from build123d import *

# Parameters (mm, degrees)
BOSS_EXTRU_1_DEPTH         = 3
CONG_1_R                   = 3
ESQUISSE2_R                = 3
PER_AGE_PROFIL_DEPTH       = 200.145675323
ESQUISSE3_R                = 1.65
PER_AGE_ENCODEUR_DEPTH     = 200.145675323
POCHE_ROUE_ENCODEUSE_DEPTH = 200.145675323
CONG_4_R                   = 1
CONG_2_R                   = 4.25
CONG_3_R                   = 4.25
ESQUISSE5_R                = 1.65
PER_AGE_BLOC_MOTEUR_DEPTH  = 200.145675323
ESQUISSE6_W                = 28
ESQUISSE6_H                = 68
POCHE_ROUE_MOTRICE_DEPTH   = 200.145675323
ESQUISSE7_R                = 3.5
PER_AGE_PATIN_DEPTH        = 200.145675323
ESQUISSE8_R                = 3
ENL_V_MAT_EXTRU_1_DEPTH    = 200.145675323
CONG_5_R                   = 6
ENL_V_MAT_EXTRU_2_REACH    = 201.146
ESQUISSE9_W                = 7.25
ESQUISSE9_H                = 65
CONG_6_R                   = 2
ESQUISSE10_R               = 1.75
ENL_V_MAT_EXTRU_3_DEPTH    = 200.145675323


with BuildPart() as part:
    # Esquisse1 → Boss.-Extru.1 (new body)
    with BuildSketch(Plane(origin=(0, 0, 0), x_dir=(1, 0, 0), z_dir=(0, 1, 0))):
        Polygon((-130, 125), (130, 125), (155, 100), (155, -100), (130, -125), (-130, -125), (-155, -100), (-155, 100), align=None)
    extrude(amount=BOSS_EXTRU_1_DEPTH)

    # Congé1
    cong_1_edges = [part.edges().sort_by_distance(p)[0] for p in [
        (155, 1.5, -100),
        (155, 1.5, 100),
        (130, 1.5, 125),
        (-130, 1.5, 125),
        (-155, 1.5, 100),
        (-155, 1.5, -100),
        (-130, 1.5, -125),
        (130, 1.5, -125),
    ]]
    fillet(cong_1_edges, radius=CONG_1_R)

    # Esquisse2 → Perçage Profilé (cut, through all)
    with BuildSketch(Plane(origin=(0, 3, 0), x_dir=(1, 0, 0), z_dir=(0, 1, 0))):
        with Locations(Location((-132, -65, 0), (0, 0, 270))):
            Circle(ESQUISSE2_R)
        with Locations(Location((-132, 65, 0), (0, 0, 90))):
            Circle(ESQUISSE2_R)
        with Locations(Location((132, -65, 0), (0, 0, 90))):
            Circle(ESQUISSE2_R)
        with Locations(Location((132, 65, 0), (0, 0, 270))):
            Circle(ESQUISSE2_R)
    extrude(amount=-PER_AGE_PROFIL_DEPTH, mode=Mode.SUBTRACT)

    # Esquisse3 → Perçage Encodeur (cut, through all)
    with BuildSketch(Plane(origin=(0, 3, 0), x_dir=(1, 0, 0), z_dir=(0, 1, 0))):
        with Locations(Location((-127, 19, 0), (0, 0, 270))):
            Circle(ESQUISSE3_R)
        with Locations(Location((-127, -19, 0), (0, 0, 270))):
            Circle(ESQUISSE3_R)
        with Locations(Location((127, -19, 0), (0, 0, 90))):
            Circle(ESQUISSE3_R)
        with Locations(Location((127, 19, 0), (0, 0, 90))):
            Circle(ESQUISSE3_R)
        with Locations(Location((-139.5, 31, 0), (0, 0, 270))):
            Circle(ESQUISSE3_R)
        with Locations(Location((-139.5, -31, 0), (0, 0, 270))):
            Circle(ESQUISSE3_R)
        with Locations(Location((139.5, -31, 0), (0, 0, 90))):
            Circle(ESQUISSE3_R)
        with Locations(Location((139.5, 31, 0), (0, 0, 90))):
            Circle(ESQUISSE3_R)
    extrude(amount=-PER_AGE_ENCODEUR_DEPTH, mode=Mode.SUBTRACT)

    # Esquisse4 → Poche Roue Encodeuse (cut, through all)
    with BuildSketch(Plane(origin=(0, 3, 0), x_dir=(1, 0, 0), z_dir=(0, 1, 0))):
        with BuildLine():
            Line((143.5, -15), (129.5, -15))
            ThreePointArc((129.5, -15), (128.792893219, -14.707106781), (128.5, -14))
            Line((128.5, -14), (128.5, 14))
            ThreePointArc((128.5, 14), (128.792893219, 14.707106781), (129.5, 15))
            Line((129.5, 15), (143.5, 15))
            Line((143.5, 15), (143.5, 32.5))
            Line((143.5, 32.5), (152, 32.5))
            Line((152, 32.5), (152, -32.5))
            Line((152, -32.5), (143.5, -32.5))
            Line((143.5, -32.5), (143.5, -15))
        make_face()
        with BuildLine():
            Line((-128.5, -14), (-128.5, 14))
            ThreePointArc((-128.5, 14), (-128.792893219, 14.707106781), (-129.5, 15))
            Line((-129.5, 15), (-143.5, 15))
            Line((-143.5, 15), (-143.5, 32.5))
            Line((-143.5, 32.5), (-152, 32.5))
            Line((-152, 32.5), (-152, -32.5))
            Line((-152, -32.5), (-143.5, -32.5))
            Line((-143.5, -32.5), (-143.5, -15))
            Line((-143.5, -15), (-129.5, -15))
            ThreePointArc((-129.5, -15), (-128.792893219, -14.707106781), (-128.5, -14))
        make_face()
    extrude(amount=-POCHE_ROUE_ENCODEUSE_DEPTH, mode=Mode.SUBTRACT)

    # Congé4
    cong_4_edges = [part.edges().sort_by_distance(p)[0] for p in [
        (-143.5, 1.5, 15),
        (-143.5, 1.5, -15),
        (143.5, 1.5, -15),
        (143.5, 1.5, 15),
    ]]
    fillet(cong_4_edges, radius=CONG_4_R)

    # Congé2
    cong_2_edges = [part.edges().sort_by_distance(p)[0] for p in [
        (-152, 1.5, 32.5),
        (-152, 1.5, -32.5),
        (152, 1.5, -32.5),
        (152, 1.5, 32.5),
    ]]
    fillet(cong_2_edges, radius=CONG_2_R)

    # Congé3
    cong_3_edges = [part.edges().sort_by_distance(p)[0] for p in [
        (143.5, 1.5, 32.5),
        (143.5, 1.5, -32.5),
        (-143.5, 1.5, 32.5),
        (-143.5, 1.5, -32.5),
    ]]
    fillet(cong_3_edges, radius=CONG_3_R - 0.0001)  # a hair under: the kernel refuses the full size

    # Esquisse5 → Perçage Bloc Moteur (cut, through all)
    with BuildSketch(Plane(origin=(0, 3, 0), x_dir=(1, 0, 0), z_dir=(0, 1, 0))):
        with Locations(Location((-88.5, 16, 0), (0, 0, 270))):
            Circle(ESQUISSE5_R)
        with Locations(Location((-88.5, -16, 0), (0, 0, 270))):
            Circle(ESQUISSE5_R)
        with Locations(Location((-36.5, -16, 0), (0, 0, 270))):
            Circle(ESQUISSE5_R)
        with Locations(Location((-36.5, 16, 0), (0, 0, 270))):
            Circle(ESQUISSE5_R)
        with Locations(Location((36.5, 16, 0), (0, 0, 90))):
            Circle(ESQUISSE5_R)
        with Locations(Location((36.5, -16, 0), (0, 0, 90))):
            Circle(ESQUISSE5_R)
        with Locations(Location((88.5, -16, 0), (0, 0, 90))):
            Circle(ESQUISSE5_R)
        with Locations(Location((88.5, 16, 0), (0, 0, 90))):
            Circle(ESQUISSE5_R)
    extrude(amount=-PER_AGE_BLOC_MOTEUR_DEPTH, mode=Mode.SUBTRACT)

    # Esquisse6 → Poche Roue Motrice (cut, through all)
    with BuildSketch(Plane(origin=(0, 3, 0), x_dir=(1, 0, 0), z_dir=(0, 1, 0))):
        with Locations((-108.5, 0)):
            Rectangle(ESQUISSE6_W, ESQUISSE6_H)
        with Locations((108.5, 0)):
            Rectangle(ESQUISSE6_W, ESQUISSE6_H)
    extrude(amount=-POCHE_ROUE_MOTRICE_DEPTH, mode=Mode.SUBTRACT)

    # Esquisse7 → Perçage Patin (cut, through all)
    with BuildSketch(Plane(origin=(0, 3, 0), x_dir=(1, 0, 0), z_dir=(0, 1, 0))):
        with Locations(Location((-130, 100, 0), (0, 0, 270))):
            Circle(ESQUISSE7_R)
        with Locations(Location((-130, -100, 0), (0, 0, 90))):
            Circle(ESQUISSE7_R)
        with Locations(Location((130, -100, 0), (0, 0, 270))):
            Circle(ESQUISSE7_R)
        with Locations(Location((130, 100, 0), (0, 0, 90))):
            Circle(ESQUISSE7_R)
    extrude(amount=-PER_AGE_PATIN_DEPTH, mode=Mode.SUBTRACT)

    # Esquisse8 → Enlèv. mat.-Extru.1 (cut, through all)
    with BuildSketch(Plane(origin=(0, 3, 0), x_dir=(1, 0, 0), z_dir=(0, 1, 0))):
        with Locations(Location((-36.5, -52, 0), (0, 0, 270))):
            Circle(ESQUISSE8_R)
        with Locations(Location((36.5, -52, 0), (0, 0, 270))):
            Circle(ESQUISSE8_R)
    extrude(amount=-ENL_V_MAT_EXTRU_1_DEPTH, mode=Mode.SUBTRACT)

    # Congé5
    cong_5_edges = [part.edges().sort_by_distance(p)[0] for p in [
        (-122.5, 1.5, 34),
        (-122.5, 1.5, -34),
        (-94.5, 1.5, -34),
        (-94.5, 1.5, 34),
        (122.5, 1.5, -34),
        (122.5, 1.5, 34),
        (94.5, 1.5, 34),
        (94.5, 1.5, -34),
    ]]
    fillet(cong_5_edges, radius=CONG_5_R)

    # Esquisse9 → Enlèv. mat.-Extru.2 (cut, up to next)
    with BuildSketch(Plane(origin=(0, 3, 0), x_dir=(1, 0, 0), z_dir=(0, 1, 0)), mode=Mode.PRIVATE) as enl_v_mat_extru_2_sk1:
        with Locations((-151.375, 0)):
            Rectangle(ESQUISSE9_W, ESQUISSE9_H)
    enl_v_mat_extru_2_tool1 = extrude(enl_v_mat_extru_2_sk1.sketch, amount=-ENL_V_MAT_EXTRU_2_REACH, mode=Mode.PRIVATE) & part.part
    # Esquisse9 → Enlèv. mat.-Extru.2 (cut, up to next)
    with BuildSketch(Plane(origin=(0, 3, 0), x_dir=(1, 0, 0), z_dir=(0, 1, 0)), mode=Mode.PRIVATE) as enl_v_mat_extru_2_sk2:
        with Locations((151.375, 0)):
            Rectangle(ESQUISSE9_W, ESQUISSE9_H)
    enl_v_mat_extru_2_tool2 = extrude(enl_v_mat_extru_2_sk2.sketch, amount=-ENL_V_MAT_EXTRU_2_REACH, mode=Mode.PRIVATE) & part.part
    add(enl_v_mat_extru_2_tool1.solids().sort_by_distance((-151.375, 3, 0))[0], mode=Mode.SUBTRACT)
    add(enl_v_mat_extru_2_tool2.solids().sort_by_distance((151.375, 3, 0))[0], mode=Mode.SUBTRACT)

    # Congé6
    cong_6_edges = [part.edges().sort_by_distance(p)[0] for p in [
        (-155, 1.5, 32.5),
        (-155, 1.5, -32.5),
        (155, 1.5, -32.5),
        (155, 1.5, 32.5),
    ]]
    fillet(cong_6_edges, radius=CONG_6_R)

    # Esquisse10 → Enlèv. mat.-Extru.3 (cut, through all)
    with BuildSketch(Plane(origin=(0, 3, 0), x_dir=(1, 0, 0), z_dir=(0, 1, 0))):
        with Locations(Location((77, 107.5, 0), (0, 0, 270))):
            Circle(ESQUISSE10_R)
        with Locations(Location((77, 87.5, 0), (0, 0, 270))):
            Circle(ESQUISSE10_R)
        with Locations(Location((-77, 87.5, 0), (0, 0, 90))):
            Circle(ESQUISSE10_R)
        with Locations(Location((-77, 107.5, 0), (0, 0, 90))):
            Circle(ESQUISSE10_R)
    extrude(amount=-ENL_V_MAT_EXTRU_3_DEPTH, mode=Mode.SUBTRACT)


solid = part.part
Geometry check sheet. Reference: the model listing, model coordinates, mm. Round coordinates to 2 decimals unless told otherwise and drop trailing zeros. Loops run counter-clockwise (first coordinate to the right, second up) from the corner with the lowest first, then second, coordinate; pieces in that order, holes last. Notation, with made-up numbers: (-15, -4.5) - (42, -4.5) arc R23 ccw to (42, 24.5) - close; hole circle Ø7 at (83.25, -16). An arc over 180 degrees is marked (long way). Answer as CSV lines item,"result".
(1) Material ranges on line 1 along Z through (x, y) = (-37, 1.6); line 2 along Z through (x, y) = (-88.5, 2.3); line 3 along X through (y, z) = (2.5, 14), recorded low to high.
Output values:
line 1,"z = -125 to -17.57, -14.43 to 14.43, 17.57 to 49.04, 54.96 to 125"
line 2,"z = -125 to -17.65, -14.35 to 14.35, 17.65 to 125"
line 3,"x = -128.5 to -122.5, -94.5 to 94.5, 122.5 to 128.5"
(2) Depth check by flat-ended pin: pin 1 Ø0.9 at (y, z) = (1.5, -1) entering from -X. Enter the tip coordinate at first touch or a pass-through.
Output values:
pin 1,"stops at x = -128.5"
(3) Cross-section at A-A, the plane x = 106.5. Enter the section's corners in (y, z).
Output values:
outline,"(0, -125) - (3, -125) - (3, -34) - (0, -34) - close; (0, 34) - (3, 34) - (3, 125) - (0, 125) - close"
(4) Release check for a two-part mould opening along X. For faces 1 (the face through (2, 3, -2)), 2 (the face through (96.304, 1.479, -32.289)), 3 (the face through (142, 1, -113)) record: released by +X, released by -X, zero draft, split by the parting line, or undercut.
Output values:
face 1,"zero draft"
face 2,"undercut"
face 3,"released by +X"
(5) Cross-section at B-B, the plane y = 2.5. Give the number of separate pieces and of enclosed holes in the cut face, and give its area (3 significant figures).
Output values:
separate pieces,"1"
enclosed holes,"32"
area,"69,600 mm²"
